from build123d import *

# Parameters (mm, degrees)
F0_W     = 88
F0_H     = 20
F0_R     = 1.75
F1_DEPTH = 3
F2_W     = 20
F2_H     = 4.5
F2_H_2   = 7.5
F3_DEPTH = 4
F6_DEPTH = 4
F4_R     = 1.75
F7_DEPTH = 25
F9_DEPTH = 3
F10_R    = 3
F11_R    = 1


# Not quite as in the source:
# - a feature names something its author has since deleted; it is built from what else it names


with BuildPart() as f1:
    # F0 (on Front) → F1 (new body)
    with BuildSketch(Plane.XZ):
        with Locations((44, -10)):
            Rectangle(F0_W, F0_H)
        with BuildLine():
            ThreePointArc((35.25, -15.5), (34.0207943633, -16.7498270258), (32.7506918489, -15.5415829716))
            ThreePointArc((32.7506918489, -15.5415829716), (32.75, -15.5), (32.7506918489, -15.4584170284))
            Line((32.7506918489, -15.4584170284), (32.7506918489, -8.0415829716))
            ThreePointArc((32.7506918489, -8.0415829716), (32.75, -8), (32.7506918489, -7.9584170284))
            ThreePointArc((32.7506918489, -7.9584170284), (34.0207943633, -6.7501729742), (35.25, -8))
            Line((35.25, -8), (35.25, -15.5))
        make_face(mode=Mode.SUBTRACT)
        with BuildLine():
            ThreePointArc((4.75, -4.2679491924), (6.1456439237, -4.6771243445), (6.75, -6))
            ThreePointArc((6.75, -6), (6.1456439237, -7.3228756555), (4.75, -7.7320508076))
            ThreePointArc((4.75, -7.7320508076), (2.75, -6), (4.75, -4.2679491924))
        make_face(mode=Mode.SUBTRACT)
        with Locations((83, -6)):
            Circle(F0_R, mode=Mode.SUBTRACT)
    extrude(amount=F1_DEPTH)

    # F2 (on face) → F3 (join)
    with BuildSketch(Plane.XZ.offset(3)):
        with Locations((45.25, -5.75)):
            Rectangle(F2_W, F2_H)
        with Locations((45.25, -11.75)):
            Rectangle(F2_W, F2_H_2)
        with Locations((45.25, -17.75)):
            Rectangle(F2_W, F2_H)
    extrude(amount=F3_DEPTH)

    # F5 (on face) → F6 (cut)
    with BuildSketch(Plane(origin=(0, 0, 0), x_dir=(-1, 0, 0), z_dir=(0, 1, 0))):
        Polygon((-43.5179491924, -4), (-46.9820508076, -4), (-48.7141016151, -7), (-46.9820508076, -10), (-43.5179491924, -10), (-41.7858983849, -7), align=None)
        Polygon((-43.5179491924, -13.5), (-46.9820508076, -13.5), (-48.7141016151, -16.5), (-46.9820508076, -19.5), (-43.5179491924, -19.5), (-41.7858983849, -16.5), align=None)
    extrude(amount=-F6_DEPTH, mode=Mode.SUBTRACT)

    # F4 (on face) → F7 (cut)
    with BuildSketch(Plane.XZ.offset(7)):
        with Locations((45.25, -7)):
            Circle(F4_R)
        with Locations((45.25, -16.5)):
            Circle(F4_R)
    extrude(amount=-F7_DEPTH, mode=Mode.SUBTRACT)

    # F8 (on face) → F9 (join)
    with BuildSketch(Plane(origin=(0, 0, -20), x_dir=(1, 0, 0), z_dir=(0, 0, -1))):
        Polygon((55.25, 3), (55.25, 7), (35.25, 7), (35.25, 3), (35.25, 0), (55.25, 0), align=None)
    extrude(amount=F9_DEPTH)

    # F10
    f10_edges = [f1.edges().sort_by_distance(p)[0] for p in [
        (35.25, -3.5, -23),
        (55.25, -3.5, -23),
    ]]
    fillet(f10_edges, radius=F10_R)

    # F11
    f11_edges = [f1.edges().sort_by_distance(p)[0] for p in [
        (44, -3, 0),
        (88, 0, -10),
        (71.625, -3, -20),
        (17.625, -3, -20),
        (0, -3, -10),
    ]]
    fillet(f11_edges, radius=F11_R)


solid = f1.part
Source: CAD feature listing. Evaluate the final solid. Frame: model axes, mm. A direction names the side the tool comes from. Give positions to 0.01 mm unless a question says otherwise; leave off trailing zeros. Write each loop counter-clockwise with the first axis right and the second up, starting at its lowest first coordinate (ties: lowest second). Pieces come first, ordered by that corner, then holes. Notation, with made-up numbers: M -12.75,85.5 L 8.25,85.5 A29 cw 8.25,114.5 Z; hole C 19,22 d3. An arc over 180 degrees is marked long. Return JSON: item names as keys, results as strings. Group by question number.
1) Cut plane C-C, the plane x = 34. Output: boundary loops of the cut face in (y, z), then the cut area to 3 significant figures.
2) Ray query, L1, parallel to Z at x = 45.25, y = -6; L2, parallel to Z at x = 4.5, y = -1.7; L3, parallel to X at y = -3.75, z = -13.25. Return the intervals inside material, ascending.
3) Cut plane D-D, the plane y = -5.75. Output: boundary loops of the cut face in (x, z), then the cut area to 3 significant figures.
4) First-contact query: pin 1 Ø2 at (x, z) = (4.5, -6) entering from -Y; pin 2 Ø0.6 at (x, y) = (77.5, -1) entering from -Z; pin 3 Ø3 at (x, z) = (19.5, -3) entering from -Y. Flat tips, straight axial feed; report the tip coordinate or a pass-through.
5) Draft query along Z for faces 1 (the face through (88, -2, -10)), 2 (the face through (54.35, -3.55, -22.14)), 3 (the face through (42.664, -1.972, -18.021)), 4 (the face through (45, -5, -3.5)). Return one class per face: released by +Z, released by -Z, zero draft, split by the parting line, or undercut.
6) Cut plane B-B, the plane z = -12.5. Output: boundary loops of the cut face in (x, y).
7) Cut plane A-A, the plane x = 45.25. Output: boundary loops of the cut face in (y, z).
8) Set-up query: faces 5 (the face through (71, -1, -20)), 6 (the face through (45, -7, -13)), 7 (the face through (32.751, -1, -12)), 8 (the face through (17, -1, -20)), 9 (the face through (47.86, -1.97, -17.98)). Return all of +Z, -Z, +X, -X, +Y, -Y with unobstructed straight access to the full face (end or side cutting, diameter ignored); none if empty.
Data:
{
 "1": {"outline": "M -3,-19 A1 ccw -2,-20 L 0,-20 L 0,-16.75 L -3,-16.75 Z; M -3,-6.75 L 0,-6.75 L 0,0 L -2,0 A1 ccw -3,-1 Z", "area": "29.6 mm²"},
 "2": {"L1": "z = -23 to -18.25, -14.75 to -8.75, -5.25 to -3.5", "L2": "z = -20 to -7.75, -4.25 to 0", "L3": "x = 35.25 to 55.25"},
 "3": {"outline": "M 35.25,-20 A3 ccw 38.25,-23 L 52.25,-23 A3 ccw 55.25,-20 L 55.25,-3.5 L 35.25,-3.5 Z; hole C 45.25,-16.5 d3.5; hole C 45.25,-7 d3.5", "area": "367 mm²"},
 "4": {"pin 1": "passes through", "pin 2": "stops at z = -20", "pin 3": "stops at y = -3"},
 "5": {"face 1": "zero draft", "face 2": "released by -Z", "face 3": "undercut", "face 4": "released by +Z"},
 "6": {"outline": "M 0,-2 A1 ccw 1,-3 L 32.75,-3 L 32.75,0 L 0,0 Z; M 35.25,-7 L 55.25,-7 L 55.25,-3 L 88,-3 L 88,-1 A1 ccw 87,0 L 35.25,0 Z"},
 "7": {"outline": "M -7,-23 L 0,-23 L 0,-19.5 L -4,-19.5 L -4,-18.25 L -7,-18.25 Z; M -7,-14.75 L -4,-14.75 L -4,-13.5 L 0,-13.5 L 0,-10 L -4,-10 L -4,-8.75 L -7,-8.75 Z; M -7,-5.25 L -4,-5.25 L -4,-4 L 0,-4 L 0,0 L -2,0 A1 ccw -3,-1 L -3,-3.5 L -7,-3.5 Z"},
 "8": {"face 5": "-Z, +X, +Y, -Y", "face 6": "+Z, -Z, +X, -X, -Y", "face 7": "+Y, -Y", "face 8": "-Z, -X, +Y, -Y", "face 9": "+Y"}
}
